```python
from build123d import *

# Parameters (mm, degrees)
SKETCH2_R                       = 24
SKETCH2_R_2                     = 21
EXTRUDE_THIN4_REACH             = 583.242
SKETCH3_R                       = 24
SKETCH3_R_2                     = 22
EXTRUDE_THIN4_DIRECTION_2_REACH = 301.813
SKETCH4_R                       = 7
CUT_EXTRUDE1_DEPTH              = 823


with BuildPart() as part:
    # Sweep-Thin1: sweep along a path in Sketch1
    with BuildLine(Plane.XY) as sweep_thin1_path:
        Line((0, 0), (0, 798))
        Line((0, 798), (-400, 798))
    # Sketch2 → Sweep-Thin1 (sweep)
    with BuildSketch(Plane(origin=(0, 0, 0), x_dir=(1, 0, 0), z_dir=(0, 1, 0))):
        Circle(SKETCH2_R)
        Circle(SKETCH2_R_2, mode=Mode.SUBTRACT)
    sweep(path=sweep_thin1_path.line, transition=Transition.RIGHT)

    # Sketch3 → Extrude-Thin4 (add, up to next)
    with BuildSketch(Plane(origin=(-399, 399, 0), x_dir=(0, 0, -1), z_dir=(0.707106781, -0.707106781, 0)), mode=Mode.PRIVATE) as extrude_thin4_sk1:
        with Locations((0, 353.781901472)):
            Circle(SKETCH3_R)
        with Locations((0, 353.781901472)):
            Circle(SKETCH3_R_2, mode=Mode.SUBTRACT)
    extrude_thin4_tool1 = extrude(extrude_thin4_sk1.sketch, amount=EXTRUDE_THIN4_REACH, mode=Mode.PRIVATE) - part.part
    add(extrude_thin4_tool1.solids().sort_by_distance((-148.838418, 649.161582, 23.321177))[0])

    # Sketch3 → Extrude-Thin4 direction 2 (add, up to next)
    with BuildSketch(Plane(origin=(-399, 399, 0), x_dir=(0, 0, -1), z_dir=(0.707106781, -0.707106781, 0)), mode=Mode.PRIVATE) as extrude_thin4_direction_2_sk1:
        with Locations((0, 353.781901472)):
            Circle(SKETCH3_R)
        with Locations((0, 353.781901472)):
            Circle(SKETCH3_R_2, mode=Mode.SUBTRACT)
    extrude_thin4_direction_2_tool1 = extrude(extrude_thin4_direction_2_sk1.sketch, amount=-EXTRUDE_THIN4_DIRECTION_2_REACH, mode=Mode.PRIVATE) - part.part
    add(extrude_thin4_direction_2_tool1.solids().sort_by_distance((-148.838418, 649.161582, 23.321177))[0])

    # Sketch4 → Cut-Extrude1 (cut, through all)
    with BuildSketch(Plane(origin=(0, 0, 0), x_dir=(1, 0, 0), z_dir=(0, 1, 0))):
        with Locations((-376.34, 0)):
            Circle(SKETCH4_R)
    extrude(amount=CUT_EXTRUDE1_DEPTH, mode=Mode.SUBTRACT)


solid = part.part
```
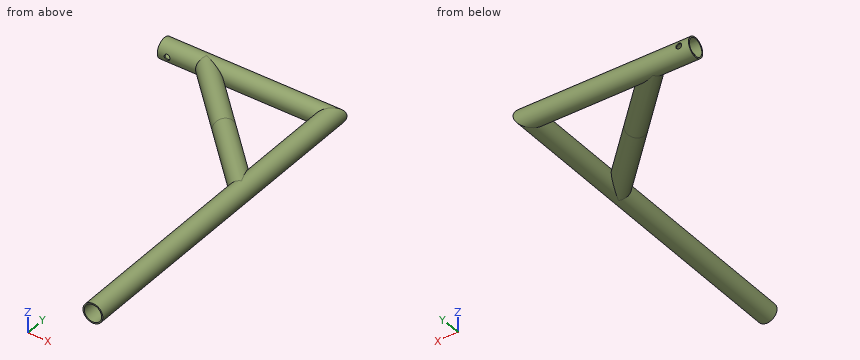
Part model, mm, in its own coordinate system. Round coordinates to 2 decimals unless told otherwise and drop trailing zeros. Order: outer loops, then holes, each group sorted by start corner. A loop starts at its lowest first (then second) coordinate and runs counter-clockwise, first axis right, second up. Notation, with made-up numbers: M -13.75,13.25 L 15.25,13.25 A14 cw 15.25,18.25 Z; hole C -22.75,-4.5 d10. An arc over 180 degrees is marked long. Answer in a Markdown table with one row per item. Add a question column.
Q1. Wall check: L1, parallel to Y at x = -279.5, z = 4; L2, parallel to Z at x = -140, y = 798; L3, parallel to Y at x = -67.5, z = 1. Give the ranges that are in metal, low to high. Write a range as from..to.
Q2. Cut at C-C on y = 681. Give the number of separate pieces and of enclosed holes in the cut face, and give its area (3 significant figures).
Q3. Cut at A-A on y = 240. Give the cut face in (x, z), and give its area (3 significant figures).
Q4. Pin check, flat tips, straight feed: pin 1 (10 mm diameter, centred on x = -143, z = 12.5, fed in from -Y); pin 2 (1 mm diameter, centred on x = -133.5, z = -11.5, fed in from -Y); pin 3 (2 mm diameter, centred on y = 706, z = -18, fed in from -X). Stop position of each tip, or through.
Q5. Cut at B-B on x = -339. Give the cut face in (y, z), and give its area (3 significant figures).
Established:
| question | item | result |
|---|---|---|
| 1 | L1 | y = 746.36..749.23, 774.34..777.38, 818.62..821.66 |
| 1 | L2 | z = -24..-21, 21..24 |
| 1 | L3 | y = 533.91..536.74, 598.9..601.73, 774.02..777.02, 818.98..821.98 |
| 2 | separate pieces | 2 |
| 2 | enclosed holes | 2 |
| 2 | area | 833 mm2 |
| 3 | outline | C 0,0 d48; hole C 0,0 d42 |
| 3 | area | 424 mm2 |
| 4 | pin 1 | stops at y = 608.13 |
| 4 | pin 2 | stops at y = 603.4 |
| 4 | pin 3 | stops at x = -229.95 |
| 5 | outline | C 798,0 d48; hole C 798,0 d42 |
| 5 | area | 424 mm2 |
